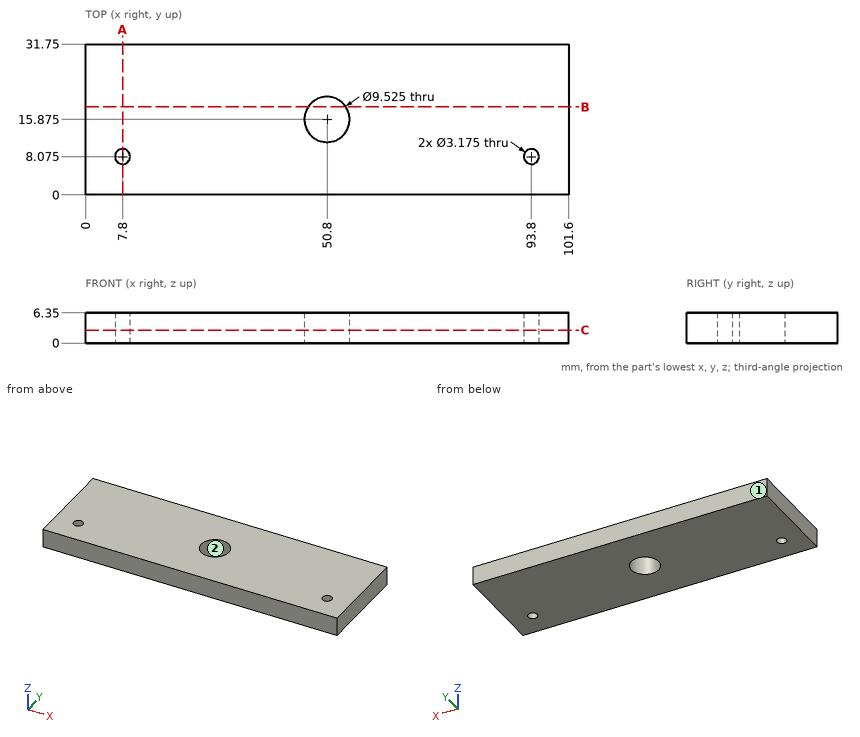
Part print with two shaded views. Sizes in mm from the minimum x, y, z corner. Coordinates: 2 decimals unless noted, no trailing zeros. Write each loop counter-clockwise with the first axis right and the second up, starting at its lowest first coordinate (ties: lowest second). Pieces come first, ordered by that corner, then holes. Notation, with made-up numbers: (-14.75, -13.5) - (37.25, -13.5) arc R21 ccw to (37.25, -3.5) - close; hole circle Ø3 at (-24.5, -40). An arc over 180 degrees is marked (long way). One line per item, written item: value. Start each with the question number.
1. Mould opens along X. For the marked faces 1 and 2 say: released by +X, released by -X, zero draft, split by the parting line, or undercut.
2. Probe line 1 (X direction, y = 15.5, z = 1); line 2 (Y direction, x = 94, z = 5.25); line 3 (Y direction, x = 55, z = 3.5). List the from-to ranges inside material, lowest first. Write a range as from..to.
3. Flat gauge pin, fed straight in: pin 1 (2 mm diameter, centred on x = 50.5, y = 18, fed in from +Z). Where does the tip first touch, or does it go through?
4. Slice it at C-C (z = 2.75). Count the separate pieces of the cut face and the enclosed holes in it, plus the area to 3 significant figures.
5. Slice it at B-B (y = 18.5). Write the cut outline in (x, z), plus the area to 3 significant figures.
6. Slice it at A-A (x = 7.8). Write the cut outline in (y, z), plus the area to 3 significant figures.
Answers below:
1. face 1: zero draft
1. face 2: undercut
2. line 1: x = 0..46.05, 55.55..101.6
2. line 2: y = 0..6.5, 9.65..31.75
2. line 3: y = 0..13.63, 18.12..31.75
3. pin 1: passes through
4. separate pieces: 1
4. enclosed holes: 3
4. area: 3,140 mm^2
5. outline: (0, 0) - (46.83, 0) - (46.83, 6.35) - (0, 6.35) - close; (54.77, 0) - (101.6, 0) - (101.6, 6.35) - (54.77, 6.35) - close
5. area: 595 mm^2
6. outline: (0, 0) - (6.49, 0) - (6.49, 6.35) - (0, 6.35) - close; (9.66, 0) - (31.75, 0) - (31.75, 6.35) - (9.66, 6.35) - close
6. area: 181 mm^2
